from build123d import *

# Parameters (mm, degrees)
SKETCH1_W           = 5
SKETCH1_H           = 19
SKETCH1_R           = 1.5
BOSS_EXTRUDE1_DEPTH = 3
FILLET1_R           = 2.5


with BuildPart() as part:
    # Sketch1 → Boss-Extrude1 (new body)
    with BuildSketch(Plane(origin=(0, 0, 0), x_dir=(1, 0, 0), z_dir=(0, 1, 0))):
        with Locations((0.46965829, 1.650333526)):
            Rectangle(SKETCH1_W, SKETCH1_H)
        with Locations(Location((0.46965829, -5.349666474, 0), (0, 0, 270))):
            Circle(SKETCH1_R, mode=Mode.SUBTRACT)
        with Locations(Location((0.46965829, 8.650333526, 0), (0, 0, 270))):
            Circle(SKETCH1_R, mode=Mode.SUBTRACT)
    extrude(amount=BOSS_EXTRUDE1_DEPTH)

    # Fillet1
    fillet1_edges = [part.edges().sort_by_distance(p)[0] for p in [
        (2.96965829, 1.5, -11.150333526),
        (-2.03034171, 1.5, -11.150333526),
        (2.96965829, 1.5, 7.849666474),
        (-2.03034171, 1.5, 7.849666474),
    ]]
    fillet(fillet1_edges, radius=FILLET1_R - 0.0001)  # a hair under: the kernel refuses the full size


solid = part.part
The model under review builds one solid part; all positions refer to its coordinate system, in mm. Round coordinates to 2 decimals unless told otherwise and drop trailing zeros. Loops run counter-clockwise (first coordinate to the right, second up) from the corner with the lowest first, then second, coordinate; pieces in that order, holes last. Notation, with made-up numbers: M 87,11 L 141,11 A16 cw 141,39 Z; hole C 11,-15.75 d9. An arc over 180 degrees is marked long. Answer as a JSON object with one key per item and string values.
Item 1: Clearance check with a flat-ended pin moving along its axis: P1, Ø2.5, axis at x = 0.47, z = -8.65, coming from the +Y side. State where the tip first meets the part, or that it passes through.
Check sheet entries:
{"P1": "through"}
Item 2: For line 1 along Z through (x, y) = (0.4, 0.75); line 2 along X through (y, z) = (2.55, -8.75), list the stretches that pass through material, from the lowest coordinate up.
Check sheet entries:
{"line 1": "-11.15 to -10.15, -7.15 to 3.85, 6.85 to 7.85", "line 2": "-2.03 to -1.03, 1.97 to 2.97"}
Item 3: We need section B-B, the plane y = 1.55. State how many separate pieces and enclosed holes the cut face has, and give its area (3 significant figures).
Check sheet entries:
{"separate pieces": "1", "enclosed holes": "2", "area": "75.5 mm2"}
Item 4: The part is to be moulded in two halves that separate along Z. For faces 1 (the face through (0.54, 1.48, 3.85)), 2 (the face through (0, 0, -2)), 3 (the face through (-1.317, 1.521, 7.098)), say which applies: +Z half, -Z half, draft (parallel to the pull), parting line (faces both ways), or undercut.
Check sheet entries:
{"face 1": "undercut", "face 2": "draft", "face 3": "+Z half"}
Item 5: We need section D-D, the plane x = -1.6. State the section outline as (y, z) points, and give its area (3 significant figures).
Check sheet entries:
{"outline": "M 0,-10.05 L 3,-10.05 L 3,6.75 L 0,6.75 Z", "area": "50.4 mm2"}
Item 6: We need section A-A, the plane x = -0.55. State the section outline as (y, z) points.
Check sheet entries:
{"outline": "M 0,-10.93 L 3,-10.93 L 3,-9.75 L 0,-9.75 Z; M 0,-7.55 L 3,-7.55 L 3,4.25 L 0,4.25 Z; M 0,6.45 L 3,6.45 L 3,7.63 L 0,7.63 Z"}
Item 7: We need section C-C, the plane x = 2.35. State the section outline as (y, z) points, and give its area (3 significant figures).
Check sheet entries:
{"outline": "M 0,-10.3 L 3,-10.3 L 3,7 L 0,7 Z", "area": "51.9 mm2"}
